```python
from build123d import *

# Parameters (mm, degrees)
SKETCH_1_W                     = 86
SKETCH_1_H                     = 86
EXTRUDE_1_DEPTH                = 12
CUT_EXTRUDE_1_DEPTH            = 2
SKETCH_3_R                     = 7
CUT_EXTRUDE_2_DEPTH            = 123.21292894
HOLE_WIZARD_M5_1_D             = 4.2
FILLET_1_R                     = 5
HOLE_WIZARD_M5_1_2_D           = 5.8
HOLE_WIZARD_M5_1_2_CBORE_D     = 10
HOLE_WIZARD_M5_1_2_CBORE_DEPTH = 7


with BuildPart() as part:
    # 草图1 → 凸台-拉伸1 (new body)
    with BuildSketch(Plane.XY):
        with Locations((43, 43)):
            Rectangle(SKETCH_1_W, SKETCH_1_H)
    extrude(amount=EXTRUDE_1_DEPTH)

    # 草图2 → 切除-拉伸1 (cut)
    with BuildSketch(Plane.XY.offset(12)):
        Polygon((71, 81), (15, 81), (15, 71), (5, 71), (5, 15), (15, 15), (15, 5), (71, 5), (71, 15), (81, 15), (81, 71), (71, 71), align=None)
    extrude(amount=-CUT_EXTRUDE_1_DEPTH, mode=Mode.SUBTRACT)

    # 草图3 → 切除-拉伸2 (cut, through all)
    with BuildSketch(Plane(origin=(0, 0, 0), x_dir=(-1, 0, 0), z_dir=(0, 0, -1))):
        with Locations((-43, 43)):
            Circle(SKETCH_3_R)
    extrude(amount=-CUT_EXTRUDE_2_DEPTH, mode=Mode.SUBTRACT)

    # Hole Wizard M5 _1 (through all)
    with Locations(Plane.XY.offset(12)):
        with Locations((77.5, 77.5), (8.5, 77.5), (8.5, 8.5), (77.5, 8.5)):
            Hole(HOLE_WIZARD_M5_1_D / 2)

    # 圆角1
    fillet_1_edges = [part.edges().sort_by_distance(p)[0] for p in [
        (15, 81, 11),
        (71, 81, 11),
        (81, 71, 11),
        (81, 15, 11),
        (71, 5, 11),
        (15, 5, 11),
        (5, 15, 11),
        (5, 71, 11),
    ]]
    fillet(fillet_1_edges, radius=FILLET_1_R)

    # Hole Wizard M5 _1 2 (through all)
    with Locations(Plane.XY.offset(12)):
        with Locations((18, 68), (68, 68), (18, 18), (68, 18)):
            CounterBoreHole(HOLE_WIZARD_M5_1_2_D / 2, HOLE_WIZARD_M5_1_2_CBORE_D / 2, HOLE_WIZARD_M5_1_2_CBORE_DEPTH)


solid = part.part
```
Input: part model. Units: mm. Frame: model coordinates. A direction names the side the tool comes from. Round coordinates to 2 decimals unless told otherwise and drop trailing zeros. Order: outer loops, then holes, each group sorted by start corner. A loop starts at its lowest first (then second) coordinate and runs counter-clockwise, first axis right, second up. Notation, with made-up numbers: (14, -12) - (24, -12) arc R17 ccw to (24, 8) - close; hole circle Ø1 at (81, 21). An arc over 180 degrees is marked (long way). Answer in a Markdown table with one row per item.
Item 1: Section query B-B (x = 68). Return the cut outline in (y, z), then the cut area to 3 significant figures.
Model answer:
| item | result |
|---|---|
| outline | (0, 0) - (15.1, 0) - (15.1, 5) - (13, 5) - (13, 10) - (5.42, 10) - (5.42, 12) - (0, 12) - close; (20.9, 0) - (65.1, 0) - (65.1, 5) - (63, 5) - (63, 10) - (23, 10) - (23, 5) - (20.9, 5) - close; (70.9, 0) - (86, 0) - (86, 12) - (80.58, 12) - (80.58, 10) - (73, 10) - (73, 5) - (70.9, 5) - close |
| area | 724 mm² |
Item 2: Reachability of faces 4 (the cylindrical face through (10.166, 76.222, 5.916)), 5 (the cylindrical face through (14, 15, 8)) from +Z, -Z, +X, -X, +Y, -Y: full face, straight path, thin tool, end or side. Return the list, or none.
Model answer:
| item | result |
|---|---|
| face 4 | +Z, -Z |
| face 5 | +Z |
Item 3: Section query C-C (z = 8.5). Give the number of separate pieces and of enclosed holes in the cut face, then the cut area to 3 significant figures.
Model answer:
| item | result |
|---|---|
| separate pieces | 1 |
| enclosed holes | 9 |
| area | 6,870 mm² |
Item 4: Mould query, pull axis Y, two halves, no side actions, for faces 1 (the flat face through (42, 86, 6)), 2 (the cylindrical face through (14, 71, 8)), 3 (the flat face through (42, 0, 6)). Classes: released by +Y, released by -Y, zero draft, split by the parting line, or undercut.
Model answer:
| item | result |
|---|---|
| face 1 | released by +Y |
| face 2 | undercut |
| face 3 | released by -Y |
Item 5: Section query A-A (y = 43). Return the cut outline in (x, z).
Model answer:
| item | result |
|---|---|
| outline | (0, 0) - (36, 0) - (36, 10) - (5, 10) - (5, 12) - (0, 12) - close; (50, 0) - (86, 0) - (86, 12) - (81, 12) - (81, 10) - (50, 10) - close |
Item 6: Pin query (flat end, axial travel): pin 1 (3 mm diameter, centred on x = 70.5, y = 67, fed in from +Z). Return the tip coordinate at first contact, or that it passes through.
Model answer:
| item | result |
|---|---|
| pin 1 | stops at z = 5 |
Item 7: Line query: line 1 (Y direction, x = 18, z = 7); line 2 (X direction, y = 23.5, z = 11.5); line 3 (Y direction, x = 68, z = 4.05). Output: solid intervals per line, ascending.
Model answer:
| item | result |
|---|---|
| line 1 | y = 0 to 13, 23 to 63, 73 to 86 |
| line 2 | x = 0 to 5, 81 to 86 |
| line 3 | y = 0 to 15.1, 20.9 to 65.1, 70.9 to 86 |
